For this review, take the finished solid that the model builds, in its own axes (mm). A direction names the side the tool comes from. Round coordinates to 2 decimals unless told otherwise and drop trailing zeros. Write each loop counter-clockwise with the first axis right and the second up, starting at its lowest first coordinate (ties: lowest second). Pieces come first, ordered by that corner, then holes. Notation, with made-up numbers: M 43,87.5 L 71,87.5 A31 cw 71,118.5 Z; hole C 40.5,9.25 d1. An arc over 180 degrees is marked long. Use one line per item in the form item = value. Start each with the question number.
Item 1: For faces 4 (the cylindrical face through (-0.104, 28.38, 28.207)), 5 (the flat face through (0, 0, 15)), 6 (the cylindrical face through (-0.028, 23.301, 28.185)), list the 3-axis set-ups (+Z, -Z, +X, -X, +Y, -Y) from which the entire face can be reached by the end or side of a thin tool; tool diameter is ignored.
Item 2: Add section C-C (y = 6). State the section outline as (x, z) points.
Item 3: Add section B-B (z = 12). State the section outline as (x, y) points.
Item 4: For P1, Ø1, axis at x = -1.5, y = 6.5, coming from the -Z side; P2, Ø0.7, axis at x = -0.5, z = -14, coming from the +Y side; P3, Ø1, axis at x = 0, z = 29, coming from the +Y side, all flat-tipped, find the tip position at first contact; note any pin that passes through.
Item 5: For line 1 (Z direction, x = -1.8, y = 26); line 2 (Z direction, x = 0, y = 28.9); line 3 (Z direction, x = -1, y = 19.5), list the stretches that pass through material, from the lowest coordinate up. Write a range as [from, to].
Item 6: Add section A-A (z = 25). State the section outline as (x, y) points, and give its area (3 significant figures).
Item 7: Draft analysis for pull direction X (two halves, no side actions). For faces 1 (the cylindrical face through (1.4, 29.8, 21)), 2 (the flat face through (2, 4, 19)), 3 (the cylindrical face through (-0.104, 28.38, 20.207)), state which applies: released by +X, released by -X, zero draft, split by the parting line, or undercut.
Item 8: Add section D-D (x = 0). Count the separate pieces of the cut face and the enclosed holes in it, and give its area (3 significant figures).
Autodesk Inventor part; units mm, degrees
ref_plane "YZ Plane" through (0, 0, 0) normal (1, 0, 0) x (0, 1, 0)
ref_plane "XZ Plane" through (0, 0, 0) normal (0, 1, 0) x (-1, 0, 0)
ref_plane "XY Plane" through (0, 0, 0) normal (0, 0, 1) x (1, 0, 0)
sketch "スケッチ1" plane through (0, 0, 0) normal (1, 0, 0) x (0, 1, 0)
  line L0 (0, 12) -> (0, -12) construction
  arc A0 (0, 0.6) -> (0, -0.6) centre (0.8, 0) ccw
  arc A1 (0, -11.4) -> (0, -12.6) centre (0.8, -12) ccw
  arc A2 (0, 12.6) -> (0, 11.4) centre (0.8, 12) ccw
  line L1 (0, 11.4) -> (0, 0.6)
  line L2 (0, -0.6) -> (0, -11.4)
  line L3 (0, -12.6) -> (0, -15)
  line L4 (0, -15) -> (-4, -15)
  line L5 (-4, -15) -> (-6, -13)
  line L6 (-6, -13) -> (-6, 26)
  line L7 (0, 32) -> (29.5, 32)
  line L8 (0, 12.6) -> (0, 17)
  line L9 (1, 18) -> (29.5, 18)
  arc A3 (1, 18) -> (0, 17) centre (1, 17) ccw
  line L10 (0.8, 12) -> (0.8, -12) construction
  arc A4 (0, 32) -> (-6, 26) centre (0, 26) ccw
  line L11 (30, 18.5) -> (30, 20.4)
  line L12 (30, 31.5) -> (29.5, 32)
  line L13 (30, 18.5) -> (29.5, 18)
  arc A5 (30, 29.6) -> (30, 28.4) centre (30.8, 29) ccw
  arc A6 (30, 21.6) -> (30, 20.4) centre (30.8, 21) ccw
  line L14 (30.8, 29) -> (30.8, 21) construction
  line L15 (30, 29.6) -> (30, 31.5)
  line L16 (30, 28.4) -> (30, 29.6) construction
  line L17 (30, 21.6) -> (30, 28.4)
  line L18 (30, 20.4) -> (30, 21.6) construction
  line L19 (30.8, 25) -> (24.681, 25) construction
  line L20 (26, 30.1) -> (24, 30.1)
  line L21 (23, 29.1) -> (23, 28.9)
  line L22 (24, 27.9) -> (26, 27.9)
  line L23 (27, 28.9) -> (27, 29.1)
  arc A7 (27, 29.1) -> (26, 30.1) centre (26, 29.1) ccw
  arc A8 (26, 27.9) -> (27, 28.9) centre (26, 28.9) ccw
  arc A9 (23, 28.9) -> (24, 27.9) centre (24, 28.9) ccw
  arc A10 (24, 30.1) -> (23, 29.1) centre (24, 29.1) ccw
  line L24 (27, 29) -> (30.8, 29) construction
  line L25 (26, 19.9) -> (24, 19.9)
  line L26 (23, 20.9) -> (23, 21.1)
  line L27 (24, 22.1) -> (26, 22.1)
  line L28 (27, 21.1) -> (27, 20.9)
  arc A11 (26, 19.9) -> (27, 20.9) centre (26, 20.9) ccw
  arc A12 (27, 21.1) -> (26, 22.1) centre (26, 21.1) ccw
  arc A13 (24, 22.1) -> (23, 21.1) centre (24, 21.1) ccw
  arc A14 (23, 20.9) -> (24, 19.9) centre (24, 20.9) ccw
  line L29 (20, 30) -> (12, 30) construction
  line L30 (12, 30) -> (12, 20) construction
  line L31 (12, 20) -> (20, 20) construction
  line L32 (20, 20) -> (20, 30) construction
  circle A15 centre (20, 30) radius 0.8
  circle A16 centre (20, 20) radius 0.8
  circle A17 centre (12, 20) radius 0.8
  circle A18 centre (12, 30) radius 0.8
  line L33 (20, 30) -> (12, 20) construction
  circle A19 centre (16, 25) radius 4
  line L34 (16, 25) -> (6, 25) construction
  circle A20 centre (6, 25) radius 4
  point P0 (0, 0)
  point P1 (0, 0)
  point P2 (30, 32)
  point P3 (30, 18)
  point P4 (27, 21)
  dimension "d0" = 24
  dimension "d1" = 1
  dimension "d2" = 0.8
  dimension "d3" = 1
  dimension "d4" = 6
  dimension "d5" = 2
  dimension "d6" = 3
  dimension "d7" = 2
  dimension "d8" = 6
  dimension "d11" = 6
  dimension "d31" = 0.5
  dimension "d32" = 0.5
  dimension "d33" = 0.5
  dimension "d34" = 0.5
  dimension "d35" = 30
  dimension "d36" = 14
  dimension "d37" = 1
  dimension "d38" = 0.8
  dimension "d39" = 8
  dimension "d40" = 1
  dimension "d41" = 3
  dimension "d42" = 4
  dimension "d43" = 2.2
  dimension "d44" = 1.6
  dimension "d45" = 10
  dimension "d46" = 8
  dimension "d47" = 10
  dimension "d48" = 10
extrude "押し出し1" add sketch "スケッチ1" along normal mid plane 4
sketch "スケッチ2" plane through (-2, 0, 11.4) normal (0, 1, 0) x (1, 0, 0)
  circle A0 centre (2, 11.4) radius 0.8
  line L0 (4, -1.2) -> (0, -1.2) construction
  line L1 (4, 0) -> (0, 0) construction
  line L2 (0, -1.2) -> (4, 0) construction
  circle A1 centre (2, -0.6) radius 0.8
  line L3 (4, 22.8) -> (0, 22.8) construction
  line L4 (4, 24) -> (0, 24) construction
  line L5 (0, 22.8) -> (4, 24) construction
  circle A2 centre (2, 23.4) radius 0.8
  dimension "d14" = 1.6
extrude "押し出し2" cut sketch "スケッチ2" against normal blind 6
sketch "スケッチ4" plane through (-2, 30, 28.4) normal (0, 1, 0) x (1, 0, 0)
  line L0 (4, -1.2) -> (0, -1.2) construction
  line L1 (4, 0) -> (0, 0) construction
  line L2 (0, -1.2) -> (4, 0) construction
  line L3 (4, 6.8) -> (0, 6.8) construction
  line L4 (4, 8) -> (0, 8) construction
  line L5 (0, 6.8) -> (4, 8) construction
  circle A0 centre (2, -0.6) radius 0.8
  circle A1 centre (2, 7.4) radius 0.8
  point P0 (2, 28.4)
  dimension "d49" = 1.6
extrude "押し出し4" cut sketch "スケッチ4" against normal blind 5
properties part number "handle"
Calculated:
q1.face_4 = +Y
q1.face_5 = -Z, +X, -X, +Y
q1.face_6 = +X, -X
q2.outline = M -2,18 L 2,18 L 2,21 L -2,21 Z; M -2,29 L 2,29 L 2,32 L -2,32 Z
q3.outline = M -2,-6 L -0.8,-6 L -0.8,-0.2 L -2,-0.2 Z; M 0.8,-6 L 2,-6 L 2,-0.2 L 0.8,-0.2 Z
q4.P1 = 18
q4.P2 = 0
q4.P3 = 23.08
q5.line_1 = [18, 19.9], [22.1, 27.9], [30.1, 32]
q5.line_2 = [18, 20.2], [21.8, 28.2], [29.8, 32]
q5.line_3 = [18, 19.38], [20.62, 23.06], [26.94, 29.38], [30.62, 32]
q6.outline = M -2,-6 L 2,-6 L 2,2 L -2,2 Z; M -2,10 L 2,10 L 2,12 L -2,12 Z; M -2,20 L 2,20 L 2,30 L -2,30 Z
q6.area = 80.0 mm^2
q7.face_1 = zero draft
q7.face_2 = released by +X
q7.face_3 = undercut
q8.separate_pieces = 4
q8.enclosed_holes = 6
q8.area = 529 mm^2
